Can you work these out from the model? Positions are in its coordinate system, mm. Face numbers are marked on the shaded views. A direction names the side the tool comes from. Round coordinates to 2 decimals unless told otherwise and drop trailing zeros. Order: outer loops, then holes, each group sorted by start corner. A loop starts at its lowest first (then second) coordinate and runs counter-clockwise, first axis right, second up. Notation, with made-up numbers: (36.25, -23) -> (90.25, -23) arc R18 ccw to (90.25, 5) -> close; hole circle Ø2 at (37.25, 57.5). An arc over 180 degrees is marked (long way). Use a Markdown table: item, result. Add a question column.
Q1. If we section it at C-C on y = 2: List the corners of the cut face in (x, z) for me, plus the area to 3 significant figures.
Q2. I'm going to push flat-ended pins straight in: pin 1 Ø22 at (x, z) = (-6.5, 6.5) entering from -Y; pin 2 Ø2.5 at (x, z) = (15.5, 0) entering from +Y; pin 3 Ø4 at (x, z) = (3.5, -11) entering from +Y; pin 4 Ø8 at (x, y) = (10.5, 2.5) entering from +Z. Where does each tip first touch, or does it pass through?
Q3. For the marked faces 1 and 2, which set-ups out of +Z, -Z, +X, -X, +Y, -Y let a thin tool reach every point of the face, with its end or its side?
Q4. If we section it at A-A on z = 0: Give the number of separate pieces and of enclosed holes in the cut face, plus the area to 3 significant figures.
Q5. I need wall thicknesses on line 1 along X through (y, z) = (-0.7, 0); line 2 along Y through (x, z) = (17, -11.5); line 3 along Z through (x, y) = (15.5, -1.1). Which ranges of each line are inside material? Lowest first, please. Write a range as [from, to].
Q6. If we section it at B-B on y = 5.25: List the corners of the cut face in (x, z) for me.
```python
from build123d import *

# Parameters (mm, degrees)
SKETCH3_R          = 2.25
CUT_EXTRUDE1_DEPTH = 12.5
FILLET1_R          = 0.5


with BuildPart() as part:
    # Sketch2 → Revolve1 (revolve)
    with BuildSketch(Plane(origin=(0, 0, 0), x_dir=(0, 0, -1), z_dir=(1, 0, 0))):
        with BuildLine():
            Line((0, 7.9375), (0, -11.0625))
            ThreePointArc((0, -11.0625), (6.296885391, -9.09550112), (10.3545, -3.894))
            ThreePointArc((10.3545, -3.894), (11.39119124, -2.565054014), (13, -2.0625))
            Line((13, -2.0625), (22.5, -2.0625))
            Line((22.5, -2.0625), (22.5, 0.4375))
            Line((22.5, 0.4375), (11.5, 0.4375))
            Line((11.5, 0.4375), (9, 3.4375))
            Line((9, 3.4375), (7.154544011, 3.4375))
            ThreePointArc((7.154544011, 3.4375), (4.226035376, 6.71896802), (0, 7.9375))
        make_face()
    revolve(axis=Axis((0, 7.9375, 0), (0, -1, 0)))

    # Sketch3 → Cut-Extrude1 (cut, through all)
    with BuildSketch(Plane(origin=(0, 0.4375, 0), x_dir=(1, 0, 0), z_dir=(0, 1, 0))):
        with Locations((-15.5, 0)):
            Circle(SKETCH3_R)
        with Locations((15.5, 0)):
            Circle(SKETCH3_R)
    extrude(amount=-CUT_EXTRUDE1_DEPTH, mode=Mode.SUBTRACT)

    # Fillet1
    fillet1_edges = [part.edges().sort_by_distance(p)[0] for p in [
        (0, 0.4375, 11.5),
        (0, 3.4375, 9),
        (0, -2.0625, 22.5),
        (0, 0.4375, 22.5),
    ]]
    fillet(fillet1_edges, radius=FILLET1_R)


solid = part.part
```
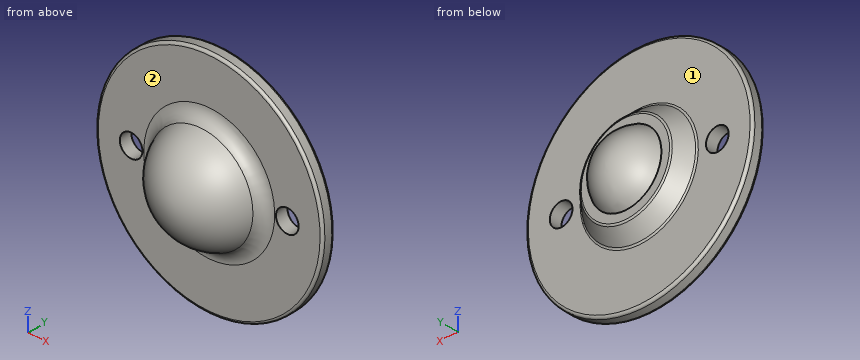
Answer below:
| question | item | result |
|---|---|---|
| 1 | outline | circle Ø20.4 at (0, 0) |
| 1 | area | 327 mm² |
| 2 | pin 1 | y = -11.06 |
| 2 | pin 2 | through |
| 2 | pin 3 | y = 2.79 |
| 2 | pin 4 | z = 21.26 |
| 3 | face 1 | +Y |
| 3 | face 2 | -Y |
| 4 | separate pieces | 3 |
| 4 | enclosed holes | 0 |
| 4 | area | 346 mm² |
| 5 | line 1 | [-22.5, -17.75], [-13.25, 13.25], [17.75, 22.5] |
| 5 | line 2 | [-2.06, 0.44] |
| 5 | line 3 | [-16.31, -2.25], [2.25, 16.31] |
| 6 | outline | circle Ø11.91 at (0, 0) |
